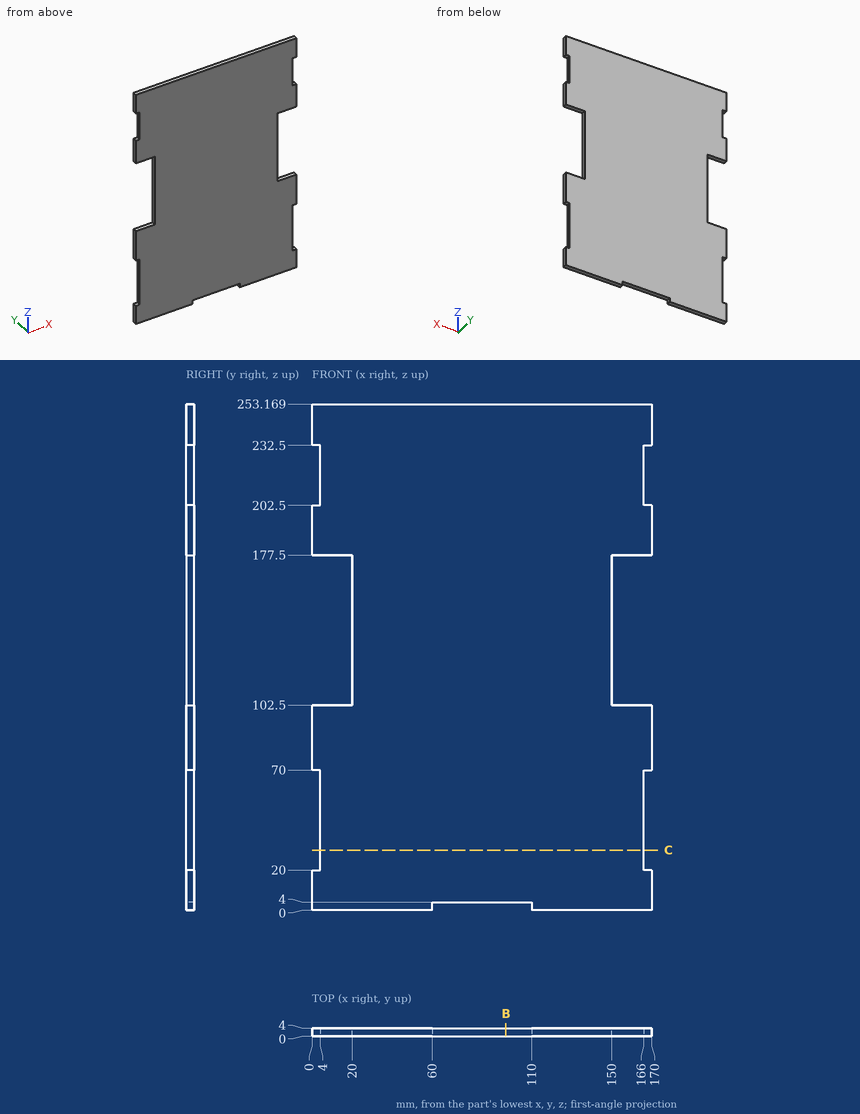
Geometry check sheet. Reference: drawing and pictorial views, mm from the part's lowest x, y, z. Give positions to 0.01 mm unless a question says otherwise; leave off trailing zeros. Order: outer loops, then holes, each group sorted by start corner. A loop starts at its lowest first (then second) coordinate and runs counter-clockwise, first axis right, second up. Notation, with made-up numbers: M 18.25,75.5 L 50.25,75.5 A31 cw 50.25,102.5 Z; hole C 13.5,22.25 d9. An arc over 180 degrees is marked long. Use one line per item in the form item = value. Start each with the question number.
Q1. Scan lines: line 1 along X through (y, z) = (1.45, 205.5); line 2 along X through (y, z) = (3.3, 133); line 3 along Z through (x, y) = (10, 2.9). Record each from-to range of solid material in increasing order. Write a range as [from, to].
Q2. Go/stop test with flat-tipped pins: pin 1 Ø1.2 at (y, z) = (2, 212) entering from -X; pin 2 Ø2 at (y, z) = (1.5, 138.5) entering from -X; pin 3 Ø2 at (y, z) = (2.5, 122.5) entering from +X. Record where each tip stops, or that it passes through.
Q3. Section check B-B (x = 97). Enter the section's corners in (y, z), then the cut area to 3 significant figures.
Q4. Section check C-C (z = 30). Enter the section's corners in (x, y).
Evaluation:
q1.line_1 = [4, 166]
q1.line_2 = [20, 150]
q1.line_3 = [0, 102.5], [177.5, 253.17]
q2.pin_1 = 4
q2.pin_2 = 20
q2.pin_3 = 150
q3.outline = M 0,4 L 4,4 L 4,253.17 L 0,253.17 Z
q3.area = 997 mm2
q4.outline = M 4,0 L 166,0 L 166,4 L 4,4 Z
